Answer from the drawing. Dimensions are ordinates in mm from the lowest x, y and z of the part. Give positions to 0.01 mm unless a question says otherwise; leave off trailing zeros. Loops run counter-clockwise (first coordinate to the right, second up) from the corner with the lowest first, then second, coordinate; pieces in that order, holes last. Notation, with made-up numbers: (79, 51) - (136, 51) arc R23 ccw to (136, 81) - close; hole circle Ø8 at (68.25, 30.25). An arc over 180 degrees is marked (long way). One line per question, with ' | ' between items. Start each with the question number.
1. Each of these flat-tipped pins is pushed along its axis until it touches: pin 1 (5 mm diameter, centred on y = 193.5, z = 4.5, fed in from +X); pin 2 (6 mm diameter, centred on x = 278.5, y = 102.5, fed in from +Z); pin 3 (3 mm diameter, centred on y = 11, z = 7, fed in from -X). Where does it stop, or does it pass through?
2. Section D-D (y = 171.5) is taken. Determine the outline of the cut face in (x, z), plus the area to 3 significant figures.
3. Section B-B (x = 28) is taken. Determine the outline of the cut face in (y, z), plus the area to 3 significant figures.
4. Section A-A (z = 4) is taken. Determine the outline of the cut face in (x, y), plus the area to 3 significant figures.
5. Section C-C (y = 128) is taken. Determine the outline of the cut face in (x, z), plus the area to 3 significant figures.
6. Find the intervals of material crossed by line 1 (X direction, y = 193, z = 7.5); line 2 (Y direction, x = 203.5, z = 3.5); line 3 (Y direction, x = 160.5, z = 1.75), in increasing order.
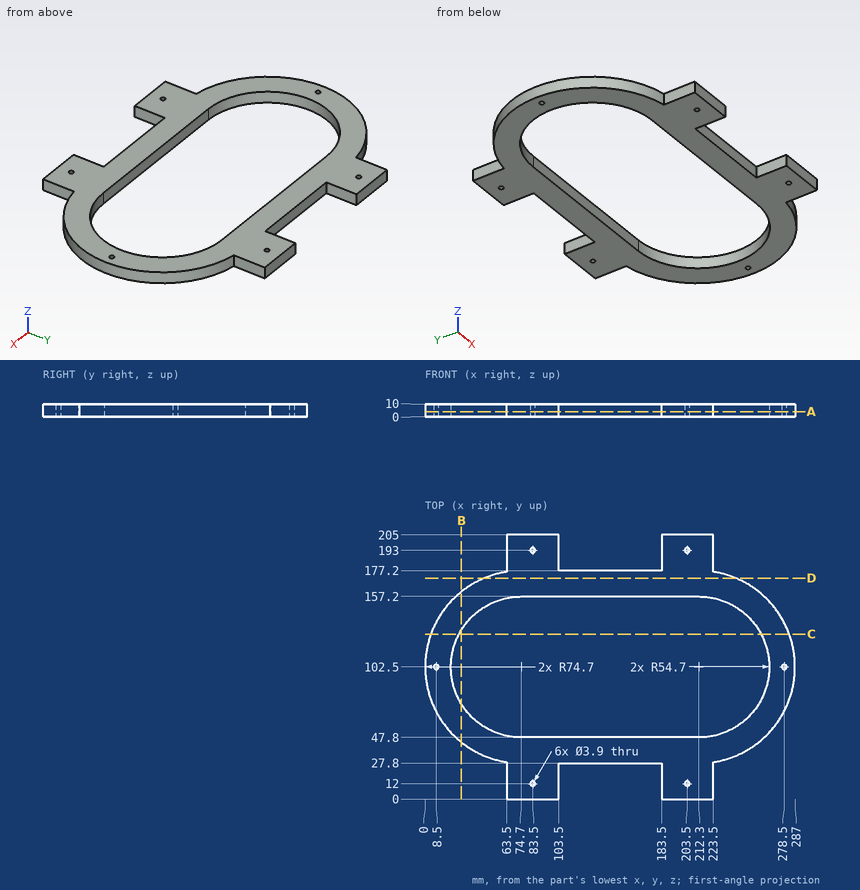
Conclusion:
1) pin 1: x = 223.5 | pin 2: z = 10 | pin 3: x = 63.5
2) outline: (46.08, 0) - (240.92, 0) - (240.92, 10) - (46.08, 10) - close | area: 1,950 mm²
3) outline: (44.2, 0) - (74.02, 0) - (74.02, 10) - (44.2, 10) - close; (130.98, 0) - (160.8, 0) - (160.8, 10) - (130.98, 10) - close | area: 596 mm²
4) outline: (63.5, 0) - (103.5, 0) - (103.5, 27.8) - (183.5, 27.8) - (183.5, 0) - (223.5, 0) - (223.5, 28.64) arc R74.7 ccw to (223.5, 176.36) - (223.5, 205) - (183.5, 205) - (183.5, 177.2) - (103.5, 177.2) - (103.5, 205) - (63.5, 205) - (63.5, 176.36) arc R74.7 ccw to (63.5, 28.64) - close; hole circle Ø3.9 at (8.5, 102.5); hole (74.7, 47.8) - (212.3, 47.8) arc R54.7 ccw to (212.3, 157.2) - (74.7, 157.2) arc R54.7 ccw to start; hole circle Ø3.9 at (83.5, 12); hole circle Ø3.9 at (83.5, 193); hole circle Ø3.9 at (203.5, 12); hole circle Ø3.9 at (203.5, 193); hole circle Ø3.9 at (278.5, 102.5) | area: 18,000 mm²
5) outline: (4.49, 0) - (26.31, 0) - (26.31, 10) - (4.49, 10) - close; (260.69, 0) - (282.51, 0) - (282.51, 10) - (260.69, 10) - close | area: 436 mm²
6) line 1: 63.5 to 81.55, 85.45 to 103.5, 183.5 to 201.55, 205.45 to 223.5 | line 2: 0 to 10.05, 13.95 to 47.8, 157.2 to 191.05, 194.95 to 205 | line 3: 27.8 to 47.8, 157.2 to 177.2
